Read the model definition and answer for the solid it produces. Units are mm, in the model's axes. Face numbers are marked on the shaded views. Give positions to 0.01 mm unless a question says otherwise; leave off trailing zeros. Write each loop counter-clockwise with the first axis right and the second up, starting at its lowest first coordinate (ties: lowest second). Pieces come first, ordered by that corner, then holes. Notation, with made-up numbers: (44, -8.75) -> (68, -8.75) arc R25 cw to (68, 11.25) -> close; hole circle Ø10 at (-32, -38.5). An arc over 180 degrees is marked (long way). Answer as CSV lines item,"result". Start each with the question number.
1. The part is cut by section B-B, the plane y = 32.5. Determine the outline of the cut face in (x, z), and give its area (3 significant figures).
2. The part is cut by section A-A, the plane z = 71. Determine the outline of the cut face in (x, y), and give its area (3 significant figures).
3. The part is cut by section D-D, the plane z = -19.5. Determine the outline of the cut face in (x, y), and give its area (3 significant figures).
4. Given pin 1 (6.5 mm diameter, centred on x = 1, y = 42, fed in from +Z); pin 2 (3 mm diameter, centred on y = 126.5, z = 62.5, fed in from +X); pin 3 (8 mm diameter, centred on x = -44, y = 41, fed in from +Z); pin 4 (9.5 mm diameter, centred on y = -19, z = -14.5, fed in from +X), each flat-ended and moving along its own axis, determine where each tip first touches the part or whether it passes through.
5. The part is cut by section C-C, the plane x = 59. Determine the outline of the cut face in (y, z).
6. For a pull along X with two mould halves and no side action, classify the marked faces 1, 2 and 3 as pulls with the +X half, pulls with the -X half, needs draft (parallel to the pull), parting line crosses it, or undercut.
7. Find the intervals of material crossed by line 1 (Z direction, x = -39.5, y = 45); line 2 (X direction, y = 22, z = -14), in increasing order.
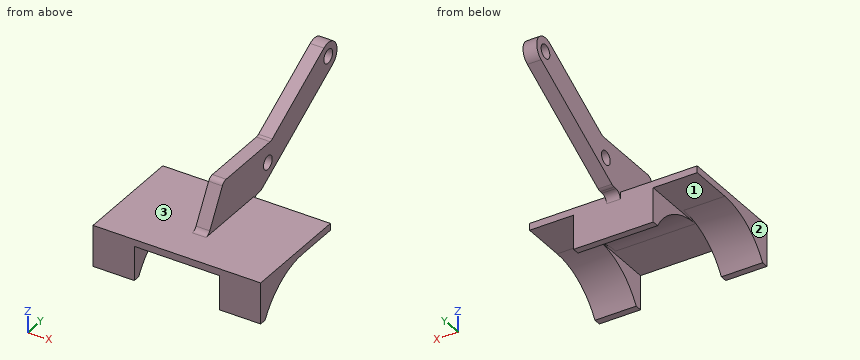
from build123d import *

# Parameters (mm, degrees)
BOSS_EXTRUDE1_DEPTH = 76.2
CUT_EXTRUDE1_DEPTH  = 38.1
BOSS_EXTRUDE5_DEPTH = 38.1
SKETCH5_R           = 6.35
BOSS_EXTRUDE6_DEPTH = 6.35
FILLET1_R           = 6.35
CUT_EXTRUDE3_DEPTH  = 2.54


with BuildPart() as part:
    # Sketch1 → Boss-Extrude1 (new body, symmetric)
    with BuildSketch(Plane(origin=(0, 0, 0), x_dir=(0, 0, -1), z_dir=(1, 0, 0))):
        with BuildLine():
            Line((0, 50.8), (38.1, 50.8))
            Line((38.1, 50.8), (38.1, 44.45))
            ThreePointArc((38.1, 44.45), (14.85738686, 21.20738686), (6.35, -10.54261314))
            Line((6.35, -10.54261314), (6.35, -50.8))
            Line((6.35, -50.8), (0, -50.8))
            Line((0, -50.8), (0, 50.8))
        make_face()
    extrude(amount=BOSS_EXTRUDE1_DEPTH, both=True)

    # Sketch6 → Cut-Extrude1 (cut)
    with BuildSketch(Plane(origin=(39.37, 0, 0), x_dir=(0, 0, -1), z_dir=(1, 0, 0))):
        with BuildLine():
            Line((0, -50.8), (6.35, -50.8))
            Line((6.35, -50.8), (6.35, -10.54261314))
            ThreePointArc((6.35, -10.54261314), (14.85738686, 21.20738686), (38.1, 44.45))
            Line((38.1, 44.45), (38.1, 50.8))
            Line((38.1, 50.8), (0, 50.8))
            Line((0, 50.8), (0, -50.8))
        make_face()
    cut_extrude1 = extrude(amount=CUT_EXTRUDE1_DEPTH, mode=Mode.SUBTRACT)

    # Mirror1: Cut-Extrude1 across plane
    add(cut_extrude1.mirror(Plane(origin=(0, 0, 0), x_dir=(0, 0, 1), z_dir=(1, 0, 0))), mode=Mode.SUBTRACT)

    # Sketch7 → Boss-Extrude5 (add)
    with BuildSketch(Plane(origin=(39.37, 0, 0), x_dir=(0, 0, -1), z_dir=(1, 0, 0))):
        with BuildLine():
            Line((0, 50.8), (0, -50.8))
            Line((0, -50.8), (38.1, -50.8))
            Line((38.1, -50.8), (38.1, -44.45))
            ThreePointArc((38.1, -44.45), (14.85738686, -21.20738686), (6.35, 10.54261314))
            Line((6.35, 10.54261314), (6.35, 50.8))
            Line((6.35, 50.8), (0, 50.8))
        make_face()
    boss_extrude5 = extrude(amount=BOSS_EXTRUDE5_DEPTH)

    # Mirror2: Boss-Extrude5 across plane
    add(boss_extrude5.mirror(Plane(origin=(0, 0, 0), x_dir=(0, 0, 1), z_dir=(1, 0, 0))))

    # Sketch5 → Boss-Extrude6 (add, symmetric)
    with BuildSketch(Plane(origin=(0, 0, 0), x_dir=(0, 0, -1), z_dir=(1, 0, 0))):
        with BuildLine():
            Line((-82.357309978, 153.382348419), (-38.1, 76.726438931))
            Line((-38.1, 76.726438931), (-38.1, 7.332348419))
            Line((-38.1, 7.332348419), (0, -14.664696837))
            Line((0, -14.664696837), (0, 14.664696837))
            Line((0, 14.664696837), (0, 61.535303163))
            Line((0, 61.535303163), (-60.360264722, 166.082348419))
            ThreePointArc((-60.360264722, 166.082348419), (-77.70878735, 170.730871047), (-82.357309978, 153.382348419))
        make_face()
        with Locations((-71.35878735, 159.732348419)):
            Circle(SKETCH5_R, mode=Mode.SUBTRACT)
        with Locations((-20.55878735, 71.744167394)):
            Circle(SKETCH5_R, mode=Mode.SUBTRACT)
    extrude(amount=BOSS_EXTRUDE6_DEPTH, both=True)

    # Fillet1
    fillet1_edges = [part.edges().sort_by_distance(p)[0] for p in [
        (0, 50.8, 0),
        (0, -14.664696837, 0),
        (0, 61.535303163, 0),
        (0, 76.726438931, 38.1),
        (0, 7.332348419, 38.1),
    ]]
    fillet(fillet1_edges, radius=FILLET1_R)

    # Sketch9 → Cut-Extrude3 (cut)
    with BuildSketch(Plane(origin=(39.37, 0, 0), x_dir=(0, 0, -1), z_dir=(1, 0, 0))):
        with BuildLine():
            Line((38.1, 50.8), (6.35, 50.8))
            Line((6.35, 50.8), (6.35, -10.54261314))
            ThreePointArc((6.35, -10.54261314), (6.570705119, -5.252921341), (7.231286278, 0))
            ThreePointArc((7.231286278, 0), (17.693368999, 25.678041777), (38.1, 44.45))
            Line((38.1, 44.45), (38.1, 50.8))
        make_face()
    cut_extrude3 = extrude(amount=-CUT_EXTRUDE3_DEPTH, mode=Mode.SUBTRACT)

    # Mirror5: Cut-Extrude3 across plane
    add(cut_extrude3.mirror(Plane(origin=(0, 0, 0), x_dir=(0, 0, 1), z_dir=(1, 0, 0))), mode=Mode.SUBTRACT)


solid = part.part
Results found:
1,outline,"(-77.47, -6.35) -> (-36.83, -6.35) -> (-36.83, -23.16) -> (36.83, -23.16) -> (36.83, -6.35) -> (77.47, -6.35) -> (77.47, 0) -> (6.35, 0) -> (6.35, 38.1) -> (-6.35, 38.1) -> (-6.35, 0) -> (-77.47, 0) -> close"
1,area,"2,710 mm²"
2,outline,"(-6.35, 133.71) -> (6.35, 133.71) -> (6.35, 153.39) -> (-6.35, 153.39) -> close; (-6.35, 166.07) -> (6.35, 166.07) -> (6.35, 172.43) -> (-6.35, 172.43) -> close"
2,area,"331 mm²"
3,outline,"(-77.47, -50.8) -> (-39.37, -50.8) -> (-39.37, -28.15) -> (-77.47, -28.15) -> close; (-36.83, 28.15) -> (36.83, 28.15) -> (36.83, 50.8) -> (-36.83, 50.8) -> close; (39.37, -50.8) -> (77.47, -50.8) -> (77.47, -28.15) -> (39.37, -28.15) -> close"
3,area,"3,390 mm²"
4,pin 1,"stops at z = 38.1"
4,pin 2,"stops at x = 6.35"
4,pin 3,"stops at z = 0"
4,pin 4,"stops at x = 77.47"
5,outline,"(-50.8, -38.1) -> (-44.45, -38.1) arc R63.5 cw to (10.54, -6.35) -> (50.8, -6.35) -> (50.8, 0) -> (-50.8, 0) -> close"
6,face 1,"undercut"
6,face 2,"pulls with the -X half"
6,face 3,"needs draft"
7,line 1,"z = -6.35 to 0"
7,line 2,"x = -36.83 to 36.83"
